from build123d import *

# Parameters (mm, degrees)
F1_R            = 77.5
F2_DEPTH        = 10
F3_R            = 2
F4_DEPTH        = 10
F4_COPIES_COUNT = 6


# Not quite as in the source:
# - a pattern or mirror of a feature is missing from the dataset's text; its kind, count and spacing are read off the source's solid


with BuildPart() as f2:
    # F1 (on Front) → F2 (new body)
    with BuildSketch(Plane.XZ):
        Circle(F1_R)
    extrude(amount=-F2_DEPTH)

    # F3
    f3_edges = [f2.edges().sort_by_distance(p)[0] for p in [
        (-77.5, 0, 0),
    ]]
    fillet(f3_edges, radius=F3_R)

    # F0 (on Front) → F4 (cut, through all)
    with BuildSketch(Plane.XZ):
        with BuildLine():
            ThreePointArc((0, 68.5), (-4.1818249581, 68.3722336919), (-8.3480500233, 67.9894113874))
            ThreePointArc((-8.3480500233, 67.9894113874), (-12.9191032665, 62.1387300384), (-7.0684219175, 57.5676767952))
            ThreePointArc((-7.0684219175, 57.5676767952), (-3.540815293, 57.8918183085), (0, 58))
            ThreePointArc((0, 58), (5.25, 63.25), (0, 68.5))
        make_face()
    f4 = extrude(amount=-F4_DEPTH, mode=Mode.SUBTRACT)

    # F4_copies: F4 ×6 about axis
    f4_copies_axis = Axis((0, 0, 0), (0, 1, 0))
    for i in range(1, F4_COPIES_COUNT):
        add(f4.rotate(f4_copies_axis, i * 360 / F4_COPIES_COUNT), mode=Mode.SUBTRACT)


solid = f2.part
Could you check a few things on this model? Use its own coordinates, in mm. Round coordinates to 2 decimals unless told otherwise and drop trailing zeros. Order: outer loops, then holes, each group sorted by start corner. A loop starts at its lowest first (then second) coordinate and runs counter-clockwise, first axis right, second up. Notation, with made-up numbers: M -12,48.25 L -2,48.25 A16 ccw -2,61.25 Z; hole C -28,49 d9. An arc over 180 degrees is marked long. One line per item, written item: value.
(1) I need wall thicknesses on line 1 along Z through (x, y) = (-55, 6); line 2 along Z through (x, y) = (56, 8); line 3 along X through (y, z) = (7.25, -58.5). Which ranges of each line are inside material? Lowest first, please. Write a range as from..to.
Ans:
line 1: z = -54.6..-40.83, -26.38..20.57, 36.87..54.6
line 2: z = -53.57..-36.73, -19.96..26.52, 39.45..53.57
line 3: x = -50.83..-2.24, 10.75..50.83
(2) I'm going to push flat-ended pins straight in: P1, Ø1, axis at y = 6.5, z = 43, coming from the -X side; P2, Ø6, axis at x = 59.5, z = -55, coming from the -Y side; P3, Ø1.5, axis at y = 5, z = -26, coming from the -X side; P4, Ø6, axis at y = 4, z = 12.5, coming from the +X side. Where does each tip first touch, or does it pass through?
Ans:
P1: stops at x = -64.81
P2: passes through
P3: stops at x = -73.27
P4: stops at x = 76.92
(3) Imagine slicing it at A-A (y = 5). Write out the boundary of the cut face in (x, z) (3 decimals), and give its area (3 significant figures).
Ans:
outline: C 0,0 d155; hole M -63.055,26.765 A5.25 ccw -53.389,22.662 A58 cw -50.229,29 A5.25 ccw -59.323,34.25 A68.5 ccw Z; hole M -59.323,-34.25 A68.5 ccw -54.707,-41.224 A5.25 ccw -46.321,-34.905 A58 cw -50.229,-29 A5.25 ccw Z; hole M -8.348,67.989 A5.25 ccw -7.068,57.568 A58 cw 0,58 A5.25 ccw 0,68.5 A68.5 ccw Z; hole M 0,-68.5 A68.5 ccw 8.348,-67.989 A5.25 ccw 7.068,-57.568 A58 cw 0,-58 A5.25 ccw Z; hole M 46.321,34.905 A58 cw 50.229,29 A5.25 ccw 59.323,34.25 A68.5 ccw 54.707,41.224 A5.25 ccw Z; hole M 50.229,-29 A5.25 ccw 59.323,-34.25 A68.5 ccw 63.055,-26.765 A5.25 ccw 53.389,-22.662 A58 cw Z
area: 17,900 mm^2
(4) If we mould it in two halves opening along Z, with no side actions, what happens to faces 1 (the flat face through (-1, 0, 1)), 2 (the cylindrical face through (52.05, 4.93, -36.11))? For each: released by +Z, released by -Z, zero draft, split by the parting line, or undercut.
Ans:
face 1: zero draft
face 2: undercut
